Build history of the part. All positions in model axes, mm. A direction names the side the tool comes from. Coordinates: 2 decimals unless noted, no trailing zeros. Write item = value, one per line. Start each with the question number.
Q1. 3-axis set-ups, long thin cutter, end or side, ignore diameter. For faces 4 (the face through (-16.69, 0.15, 326.4)), 5 (the face through (0, 0, 0)), 6 (the face through (-23.31, 0.15, 7.6)): which of +Z, -Z, +X, -X, +Y, -Y reach the whole face in a straight line?
Q2. Drill centre lines: probe 1 along Z at (x, y) = (9, 1.5); probe 2 along X at (y, z) = (0, 7); probe 3 along X at (y, z) = (2.75, 155). Where is each one in solid material? Low to high.
Q3. Pull direction X, two halves, no side cores. Call faces 1 (the face through (0, -5.35, 165)), 2 (the face through (-27.5, 0, 165)), 3 (the face through (16.69, 0.15, 7.6)): released by +X, released by -X, zero draft, split by the parting line, or undercut.
Q4. Pin check, flat tips, straight feed: P1, Ø3.5, axis at x = -9, z = 155, coming from the -Y side; P2, Ø5.5, axis at x = 9, z = 155, coming from the -Y side; P3, Ø4, axis at x = 20, y = 0, coming from the -Z side. Stop position of each tip, or through.
```python
from build123d import *

# Parameters (mm, degrees)
ESBO_O1_W                                   = 55
ESBO_O1_H                                   = 10.7
RESSALTO_EXTRUS_O1_DEPTH                    = 334
FURO_ROSCADO_PARA_CONDU_TE_DE_M4X0_71_D     = 4.2
FURO_ROSCADO_PARA_CONDU_TE_DE_1_4_281_D     = 6.6294
FURO_ROSCADO_PARA_CONDU_TE_DE_1_4_281_DEPTH = 15
FURO_ROSCADO_PARA_CONDU_TE_DE_1_4_281_TIP   = 1.991672694
FURO_ROSCADO_PARA_CONDU_TE_DE_1_4_282_D     = 6.6294
FURO_ROSCADO_PARA_CONDU_TE_DE_1_4_282_DEPTH = 15
FURO_ROSCADO_PARA_CONDU_TE_DE_1_4_282_TIP   = 1.991672694


with BuildPart() as part:
    # Esboço1 → Ressalto-extrusão1 (new body)
    with BuildSketch(Plane.XY):
        Rectangle(ESBO_O1_W, ESBO_O1_H)
    extrude(amount=RESSALTO_EXTRUS_O1_DEPTH)

    # Furo roscado para conduíte de M4x0.71 (through all)
    with Locations(Plane(origin=(0, -5.35, 0), x_dir=(-1, 0, 0), z_dir=(0, -1, 0))):
        with Locations((9, -155), (-9, -155), (-9, -179), (9, -179)):
            Hole(FURO_ROSCADO_PARA_CONDU_TE_DE_M4X0_71_D / 2)

    # Furo roscado para conduíte de 1/4-281
    with Locations(Plane.XY.offset(334)):
        with Locations((-20, 0), (20, 0)):
            Hole(FURO_ROSCADO_PARA_CONDU_TE_DE_1_4_281_D / 2, depth=FURO_ROSCADO_PARA_CONDU_TE_DE_1_4_281_DEPTH)
            with Locations((0, 0, -(FURO_ROSCADO_PARA_CONDU_TE_DE_1_4_281_DEPTH + FURO_ROSCADO_PARA_CONDU_TE_DE_1_4_281_TIP / 2))):  # 118° drill point
                Cone(0, FURO_ROSCADO_PARA_CONDU_TE_DE_1_4_281_D / 2, FURO_ROSCADO_PARA_CONDU_TE_DE_1_4_281_TIP, mode=Mode.SUBTRACT)

    # Furo roscado para conduíte de 1/4-282
    with Locations(Plane(origin=(0, 0, 0), x_dir=(-1, 0, 0), z_dir=(0, 0, -1))):
        with Locations((-20, 0), (20, 0)):
            Hole(FURO_ROSCADO_PARA_CONDU_TE_DE_1_4_282_D / 2, depth=FURO_ROSCADO_PARA_CONDU_TE_DE_1_4_282_DEPTH)
            with Locations((0, 0, -(FURO_ROSCADO_PARA_CONDU_TE_DE_1_4_282_DEPTH + FURO_ROSCADO_PARA_CONDU_TE_DE_1_4_282_TIP / 2))):  # 118° drill point
                Cone(0, FURO_ROSCADO_PARA_CONDU_TE_DE_1_4_282_D / 2, FURO_ROSCADO_PARA_CONDU_TE_DE_1_4_282_TIP, mode=Mode.SUBTRACT)


solid = part.part
```
Recorded:
q1.face_4 = +Z
q1.face_5 = -Z, +X, -X, +Y, -Y
q1.face_6 = -Z
q2.probe_1 = 0 to 152.9, 157.1 to 176.9, 181.1 to 334
q2.probe_2 = -27.5 to -23.31, -16.69 to 16.69, 23.31 to 27.5
q2.probe_3 = -27.5 to -11.1, -6.9 to 6.9, 11.1 to 27.5
q3.face_1 = zero draft
q3.face_2 = released by -X
q3.face_3 = undercut
q4.P1 = through
q4.P2 = -5.35
q4.P3 = 15.79
